from build123d import *

# Parameters (mm, degrees)
BOSS_EXTRUDE1_DEPTH     = 10.6
FILLET4_SIZE            = 4.5
FILLET4_SIZE_2          = 7.5
FILLET3_SIZE            = 7.5
FILLET3_SIZE_2          = 4.5
FILLET5_START           = -47
FILLET5_DEPTH           = 146
FILLET6_START           = -47
FILLET6_DEPTH           = 146
CUT_EXTRUDE1_DEPTH      = 0.0001
CUT_EXTRUDE1_DEPTH_BACK = 47.330240243
USB_OUTPUT_W            = 13.1
USB_OUTPUT_H            = 5.5
CUT_EXTRUDE2_DEPTH      = 11.5
BOSS_EXTRUDE2_DEPTH     = 0.7
SKETCH6_R               = 0.5
CUT_EXTRUDE3_DEPTH      = 0.01
SKETCH8_R               = 0.5
CUT_EXTRUDE4_DEPTH      = 0.01
SKETCH9_R               = 0.5
CUT_EXTRUDE5_DEPTH      = 0.01
SKETCH11_R              = 0.5
CUT_EXTRUDE7_DEPTH      = 0.01


with BuildPart() as part:
    # Sketch1 → Boss-Extrude1 (new body)
    with BuildSketch(Plane(origin=(0, 0, 0), x_dir=(1, 0, 0), z_dir=(0, 1, 0))):
        with BuildLine():
            Line((-38.762171266, 45.621027844), (90.737828734, 45.621027844))
            ThreePointArc((90.737828734, 45.621027844), (96.041129593, 43.424328703), (98.237828734, 38.121027844))
            Line((98.237828734, 38.121027844), (98.237828734, -17.778972156))
            ThreePointArc((98.237828734, -17.778972156), (96.041129593, -23.082273015), (90.737828734, -25.278972156))
            Line((90.737828734, -25.278972156), (-38.762171266, -25.278972156))
            ThreePointArc((-38.762171266, -25.278972156), (-44.065472124, -23.082273015), (-46.262171266, -17.778972156))
            Line((-46.262171266, -17.778972156), (-46.262171266, 38.121027844))
            ThreePointArc((-46.262171266, 38.121027844), (-44.065472124, 43.424328703), (-38.762171266, 45.621027844))
        make_face()
    extrude(amount=BOSS_EXTRUDE1_DEPTH)

    # Fillet4
    # a fillet whose section is not a circle: 7.5, 4.5 mm, written as the material it takes off along each edge
    with BuildSketch(Plane(origin=(109.487828734, 0, 25.278972156), x_dir=(0, 1, 0), z_dir=(-1, 0, 0))) as fillet4_piece_1:
        with BuildLine():
            Bezier((FILLET4_SIZE, 0), (0, 0), (0, FILLET4_SIZE_2), weights=[1, 0.707106781, 1])
            Line((0, FILLET4_SIZE_2), (0, 0))
            Line((0, 0), (FILLET4_SIZE, 0))
        make_face()
    extrude(amount=167, mode=Mode.SUBTRACT)

    # Fillet3
    # a fillet whose section is not a circle: 7.5, 4.5 mm, written as the material it takes off along each edge
    with BuildSketch(Plane(origin=(109.487828734, 10.6, 25.278972156), x_dir=(0, 0, -1), z_dir=(-1, 0, 0))) as fillet3_piece_1:
        with BuildLine():
            Bezier((FILLET3_SIZE, 0), (0, 0), (0, FILLET3_SIZE_2), weights=[1, 0.707106781, 1])
            Line((0, FILLET3_SIZE_2), (0, 0))
            Line((0, 0), (FILLET3_SIZE, 0))
        make_face()
    extrude(amount=167, mode=Mode.SUBTRACT)

    # Fillet5: read off the stored shape, not the designer's step
    # Fillet5 outline → Fillet5 (cut)
    with BuildSketch(Plane.YZ.offset(FILLET5_START)):
        with BuildLine():
            Line((10.6, -45.621027844), (10.6, -38.121027844))
            add(Edge.make_bspline(
                [(10.6, -38.121027844), (10.6, -45.621027844), (6.1, -45.621027844)],
                knots=[0, 0, 0, 1, 1, 1], degree=2, weights=[1, 0.707106781, 1]))
            Line((6.1, -45.621027844), (10.6, -45.621027844))
        make_face()
    extrude(amount=FILLET5_DEPTH, mode=Mode.SUBTRACT)

    # Fillet6: read off the stored shape, not the designer's step
    # Fillet6 outline → Fillet6 (cut)
    with BuildSketch(Plane.YZ.offset(FILLET6_START)):
        with BuildLine():
            Line((0, -45.621027844), (4.5, -45.621027844))
            add(Edge.make_bspline(
                [(4.5, -45.621027844), (0, -45.621027844), (0, -38.121027844)],
                knots=[0, 0, 0, 1, 1, 1], degree=2, weights=[1, 0.707106781, 1]))
            Line((0, -38.121027844), (0, -45.621027844))
        make_face()
    extrude(amount=FILLET6_DEPTH, mode=Mode.SUBTRACT)

    # USB Output → Cut-Extrude1 (cut, two sides: drawn at the far end of the back side and taken through both)
    with BuildSketch(Plane(origin=(0, 0, -28.925486843), x_dir=(0, 0, -1), z_dir=(1, 0, 0)).offset(-CUT_EXTRUDE1_DEPTH_BACK)):
        with Locations((2.092448173, 5.540415323)):
            Rectangle(USB_OUTPUT_W, USB_OUTPUT_H)
    extrude(amount=CUT_EXTRUDE1_DEPTH + CUT_EXTRUDE1_DEPTH_BACK, mode=Mode.SUBTRACT)

    # USB Charger → Cut-Extrude2 (cut)
    with BuildSketch(Plane.ZY.offset(46.262171266)):
        with BuildLine():
            Line((-18.574888724, 6.232091877), (-13.974888724, 6.232091877))
            ThreePointArc((-13.974888724, 6.232091877), (-12.914228552, 5.792752049), (-12.474888724, 4.732091877))
            Line((-12.474888724, 4.732091877), (-12.474888724, 4.132091877))
            Line((-12.474888724, 4.132091877), (-20.074888724, 4.132091877))
            Line((-20.074888724, 4.132091877), (-20.074888724, 4.732091877))
            ThreePointArc((-20.074888724, 4.732091877), (-19.635548896, 5.792752049), (-18.574888724, 6.232091877))
        make_face()
    extrude(amount=-CUT_EXTRUDE2_DEPTH, mode=Mode.SUBTRACT)

    # Sketch4 → Boss-Extrude2 (add)
    with BuildSketch(Plane.ZY.offset(46.262171266)):
        with BuildLine():
            Line((18.15777008, 6.213830992), (11.65777008, 6.213830992))
            ThreePointArc((11.65777008, 6.213830992), (11.021373976, 5.950227095), (10.75777008, 5.313830992))
            Line((10.75777008, 5.313830992), (10.75777008, 5.113830992))
            ThreePointArc((10.75777008, 5.113830992), (11.021373976, 4.477434889), (11.65777008, 4.213830992))
            Line((11.65777008, 4.213830992), (18.15777008, 4.213830992))
            ThreePointArc((18.15777008, 4.213830992), (18.794166183, 4.477434889), (19.05777008, 5.113830992))
            Line((19.05777008, 5.113830992), (19.05777008, 5.313830992))
            ThreePointArc((19.05777008, 5.313830992), (18.794166183, 5.950227095), (18.15777008, 6.213830992))
        make_face()
    extrude(amount=BOSS_EXTRUDE2_DEPTH)

    # Sketch6 → Cut-Extrude3 (cut)
    with BuildSketch(Plane(origin=(-46.262171266, 0, -7.484845673), x_dir=(0, 0, 1), z_dir=(-1, 0, 0))):
        with Locations((8.355271575, 5.224549503)):
            Circle(SKETCH6_R)
    extrude(amount=-CUT_EXTRUDE3_DEPTH, mode=Mode.SUBTRACT)

    # Sketch8 → Cut-Extrude4 (cut)
    with BuildSketch(Plane.ZY.offset(46.262171266)):
        with Locations((8.346381579, 5.258350764)):
            Circle(SKETCH8_R)
    extrude(amount=-CUT_EXTRUDE4_DEPTH, mode=Mode.SUBTRACT)

    # Sketch9 → Cut-Extrude5 (cut)
    with BuildSketch(Plane(origin=(-46.262171266, 1.999999249, 4.454543781), x_dir=(0, 0, 1), z_dir=(-1, 0, 0))):
        with Locations((1.386907241, 3.201460838)):
            Circle(SKETCH9_R)
    extrude(amount=-CUT_EXTRUDE5_DEPTH, mode=Mode.SUBTRACT)

    # Sketch11 → Cut-Extrude7 (cut)
    with BuildSketch(Plane(origin=(-46.262171266, 2.666665665, -5.363634349), x_dir=(0, 0, 1), z_dir=(-1, 0, 0))):
        with Locations((8.659631782, 2.56509744)):
            Circle(SKETCH11_R)
    extrude(amount=-CUT_EXTRUDE7_DEPTH, mode=Mode.SUBTRACT)


solid = part.part
For this review, take the finished solid that the model builds, in its own axes (mm). A direction names the side the tool comes from. Coordinates: 2 decimals unless noted, no trailing zeros. Write each question's results on one line, items separated by ' | '. Start each with the question number.
1) Insertion check: pin 1 (5 mm diameter, centred on y = 2.5, z = -4.5, fed in from -X). The pin has a flat end and moves straight along its axis. Give the tip position at first contact, or say it passes through.
2) Wall thickness on L1, parallel to Y at x = -4.5, z = -27.5; L2, parallel to X at y = 6.75, z = -22; L3, parallel to X at y = 7, z = -27.5: over which ranges is each line inside the solid? List them lowest first. Write a range as [from, to].
3) For faces 5 (the face through (27, 10.6, -11)), 6 (the face through (0, 6, -31)), list the 3-axis set-ups (+Z, -Z, +X, -X, +Y, -Y) from which the entire face can be reached by the end or side of a thin tool; tool diameter is ignored.
4) The part is to be moulded in two halves that separate along Z. For faces 1 (the face through (-41, 4.132, -16)), 2 (the face through (-23, 8.29, -31)), 3 (the face through (96.834, 5.226, -42.49)), 4 (the face through (96.93, 5.23, 22.01)), say which applies: +Z half, -Z half, draft (parallel to the pull), parting line (faces both ways), or undercut.
Geometry says:
1) pin 1: x = -46.26
2) L1: [0, 2.79], [8.29, 10.6] | L2: [-46.26, 98.24] | L3: [0, 98.24]
3) face 5: +Z, -Z, +X, -X, +Y | face 6: -X
4) face 1: undercut | face 2: undercut | face 3: -Z half | face 4: +Z half
